Input: part model. Units: mm. Frame: model coordinates. A direction names the side the tool comes from. Coordinates: 2 decimals unless noted, no trailing zeros. Loops run counter-clockwise (first coordinate to the right, second up) from the corner with the lowest first, then second, coordinate; pieces in that order, holes last.
(1) Line query: L1, parallel to Y at x = 0, z = 18.95; L2, parallel to X at y = 20.5, z = 6.25; L3, parallel to X at y = -16, z = 4. Output: solid intervals per line, ascending.
(2) Mould query, pull axis Z, two halves, no side actions, for faces 4 (the face through (-5.405, -24.339, 1.875)), 5 (the face through (25.28, -0.59, 5.1)), 6 (the face through (23.846, 7.509, 15.07)). Classes: released by +Z, released by -Z, zero draft, split by the parting line, or undercut.
(3) Contact query for flat-ended pins moving along their axis: P1, Ø4, axis at x = -6.5, z = 10, coming from the +Y side; P2, Ø1.5, axis at y = 2.5, z = 3.5, coming from the +X side; P3, Ø5, axis at y = -6, z = 14, coming from the +X side; P4, Ø8, axis at x = 15.5, y = 10.5, coming from the +Z side. Output: stop coordinate, or through.
(4) Section A-A, the plane z = 16.5. Return loops of the section in (x, y), then the cut area to 3 significant figures.
(5) Set-up query: faces 1 (the face through (-0.02, 27.95, 1.75)), 2 (the face through (10.382, -19.961, 18.986)), 3 (the face through (-22.34, 3.82, 20)). Return all of +Z, -Z, +X, -X, +Y, -Y with unobstructed straight access to the full face (end or side cutting, diameter ignored); none if empty.
(6) Section B-B, the plane z = 3. Return loops of the section in (x, y).
```python
from build123d import *

# Parameters (mm, degrees)
F4_D            = 2.5781
F4_COPIES_COUNT = 3
F7_W            = 1.5
F7_H            = 2
F8_DEPTH        = 25


# Not quite as in the source:
# - a pattern or mirror of a feature is missing from the dataset's text; its kind, count and spacing are read off the source's solid


with BuildPart() as f1:
    # F0 (on Front) → F1 (revolve)
    with BuildSketch(Plane.XZ):
        Polygon((22.5, 18), (20, 18), (20, 10), (21.8094010768, 6.8660254038), (22.3094010768, 6), (24.6188021535, 2), (29.6188021535, 0), (29.6188021535, 2), (25, 10), (25, 18), (25, 20), (22.5, 20), align=None)
    revolve(axis=Axis((0, 0, 41.8434557322), (0, 0, 1)))

    # F4 (through all)
    with Locations(Plane(origin=(23.0801270189, 0, 13.3253175473), x_dir=(0, 1, 0), z_dir=(0.8660254038, 0, 0.5))):
        with Locations((0, -7.0773502692)):
            f4 = Hole(F4_D / 2)

    # F4_copies: F4 ×3 about axis
    f4_copies_axis = Axis((0, 0, 0), (0, 0, 1))
    for i in range(1, F4_COPIES_COUNT):
        add(f4.rotate(f4_copies_axis, i * 360 / F4_COPIES_COUNT), mode=Mode.SUBTRACT)

    # F7 (on line) → F8 (cut)
    with BuildSketch(Plane(origin=(0, 29.619, 0), x_dir=(-1, 0, 0), z_dir=(0, 1, 0))):
        Rectangle(F7_W, F7_H)
        with BuildLine():
            Line((-0.75, 1), (0.75, 1))
            ThreePointArc((0.75, 1), (0, 1.75), (-0.75, 1))
        make_face()
    extrude(amount=-F8_DEPTH, mode=Mode.SUBTRACT)


solid = f1.part
```
Report:
1. L1: y = -25 to -22.5, 22.5 to 25
1. L2: x = -17.82 to -13.29, -10.79 to -8.43, 8.43 to 17.82
1. L3: x = -23.54 to -17.16, 17.16 to 23.54
2. face 4: released by -Z
2. face 5: undercut
2. face 6: zero draft
3. P1: stops at y = 25.43
3. P2: stops at x = 29.08
3. P3: stops at x = 24.75
3. P4: stops at z = 20
4. outline: circle Ø50 at (0, 0); hole circle Ø40 at (0, 0)
4. area: 707 mm2
5. face 1: -Z, +Y
5. face 2: +Z
5. face 3: +Z, +X, -X, +Y, -Y
6. outline: circle Ø58.08 at (0, 0); hole circle Ø48.08 at (0, 0)
